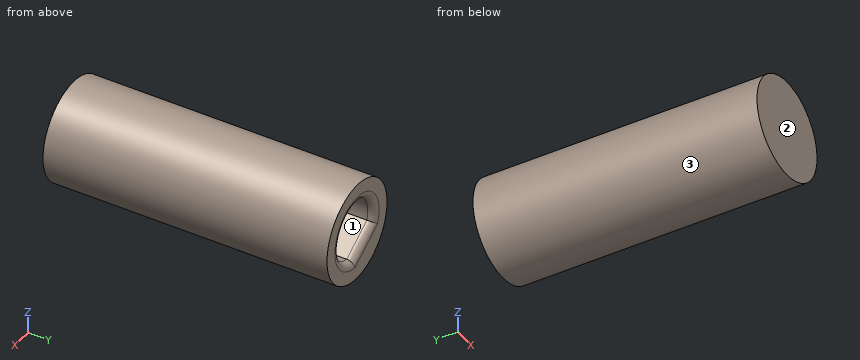
```python
from build123d import *

# Parameters (mm, degrees)
SKETCH1_R           = 7
BOSS_EXTRUDE1_DEPTH = 40
FILLET1_R           = 1
SKETCH2_R           = 4.15
BOSS_EXTRUDE2_DEPTH = 10


with BuildPart() as part:
    # Sketch1 → Boss-Extrude1 (new body)
    with BuildSketch(Plane(origin=(0, 0, 0), x_dir=(1, 0, 0), z_dir=(0, 1, 0))):
        with Locations(Location((0, 0, 0), (0, 0, 270))):
            Circle(SKETCH1_R)
        with BuildLine():
            Line((-3.967096862, 1.218459063), (0.726242752, 4.085960287))
            ThreePointArc((0.726242752, 4.085960287), (2.163660014, -3.541338072), (-3.967096862, 1.218459063))
        make_face(mode=Mode.SUBTRACT)
    extrude(amount=BOSS_EXTRUDE1_DEPTH)

    # Fillet1
    fillet1_edges = [part.edges().sort_by_distance(p)[0] for p in [
        (-1.620427055, 40, -2.652209675),
        (2.163660014, 40, 3.541338072),
    ]]
    fillet(fillet1_edges, radius=FILLET1_R)

    # Sketch2 → Boss-Extrude2 (add)
    with BuildSketch(Plane.XZ):
        Circle(SKETCH2_R)
    extrude(amount=-BOSS_EXTRUDE2_DEPTH)


solid = part.part
```
Design review of the part built by this model. Coordinates are the model's own, in mm. Face numbers are marked on the shaded views. Coordinates: 2 decimals unless noted, no trailing zeros. Order: outer loops, then holes, each group sorted by start corner. A loop starts at its lowest first (then second) coordinate and runs counter-clockwise, first axis right, second up. Notation, with made-up numbers: (72.5, -31.5) -> (86.5, -31.5) arc R29 cw to (86.5, 0.5) -> close; hole circle Ø5 at (76, -27). An arc over 180 degrees is marked (long way). One line per item, written item: value. Start each with the question number.
Q1. Take a section at A-A, the plane y = 10.5. State the section outline as (x, z) points.
Q2. For probe 1 along X at (y, z) = (24, 0); probe 2 along Y at (x, z) = (-2.75, 0); probe 3 along Z at (x, y) = (-0.5, 26), list the stretches that pass through material, from the lowest coordinate up.
Q3. Insertion check: pin 1 Ø1 at (y, z) = (9.5, 0.5) entering from -X; pin 2 Ø2 at (x, y) = (-5, 28.5) entering from +Z; pin 3 Ø1.5 at (y, z) = (30.5, -5.5) entering from +X; pin 4 Ø6.5 at (x, z) = (0, -0.5) entering from +Y. Each pin has a flat end and moves straight along its axis. Give the tip position at first contact, or say it passes through.
Q4. Mouldability with a two-part tool opening along X and no side actions: class the marked faces 1, 2 and 3 as pulls with the +X half, pulls with the -X half, needs draft (parallel to the pull), parting line crosses it, or undercut.
Values follow:
1. outline: circle Ø14 at (0, 0); hole (-3.97, -1.22) -> (0.73, -4.09) arc R4.15 ccw (long way) to start
2. probe 1: x = -7 to -4.15, 4.15 to 7
2. probe 2: y = 0 to 10
2. probe 3: z = -6.98 to -3.34, 4.12 to 6.98
3. pin 1: stops at x = -7
3. pin 2: stops at z = 5.74
3. pin 3: stops at x = 5.14
3. pin 4: stops at y = 39.9
4. face 1: undercut
4. face 2: needs draft
4. face 3: parting line crosses it
